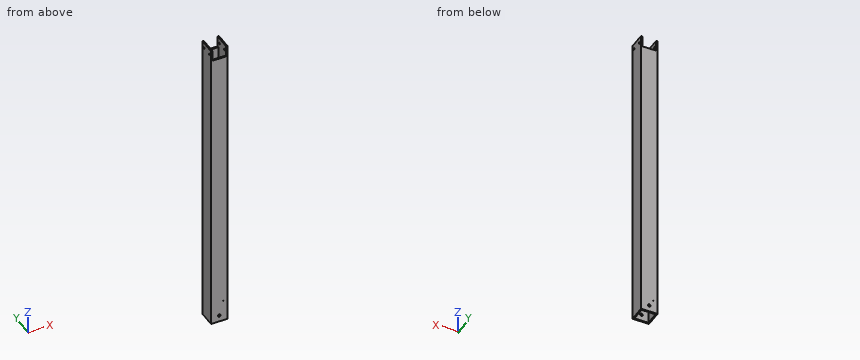
```python
from build123d import *

# Parameters (mm, degrees)
ESQUISSE2_W             = 38.1
ESQUISSE2_H             = 38.1
ESQUISSE2_W_2           = 31.75
ESQUISSE2_H_2           = 31.75
BOSS_EXTRU_1_DEPTH      = 350
ESQUISSE3_R             = 2.159
ENL_V_MAT_EXTRU_1_DEPTH = 353.582632159
ESQUISSE4_W             = 31.75
ESQUISSE4_H             = 25.4
ENL_V_MAT_EXTRU_2_DEPTH = 353.582632159
ESQUISSE6_R             = 3.175
ENL_V_MAT_EXTRU_3_DEPTH = 353.582632159
ESQUISSE8_R             = 0.5
ENL_V_MAT_EXTRU_4_DEPTH = 352.035332979
ESQUISSE8_3_R           = 0.5
ENL_V_MAT_EXTRU_5_DEPTH = 352.035332979


with BuildPart() as part:
    # Esquisse2 → Boss.-Extru.1 (new, symmetric)
    with BuildSketch(Plane.XY):
        Rectangle(ESQUISSE2_W, ESQUISSE2_H)
        Rectangle(ESQUISSE2_W_2, ESQUISSE2_H_2, mode=Mode.SUBTRACT)
    extrude(amount=BOSS_EXTRU_1_DEPTH, both=True)

    # Esquisse3 → Enl_v. mat.-Extru.1 (cut, through all)
    with BuildSketch(Plane.ZY.offset(19.05)):
        with Locations((337.3, -11.43)):
            Circle(ESQUISSE3_R)
    enl_v_mat_extru_1 = extrude(amount=-ENL_V_MAT_EXTRU_1_DEPTH, mode=Mode.SUBTRACT)

    # Sym_trie1: Enl_v. mat.-Extru.1 across plane
    add(enl_v_mat_extru_1.mirror(Plane.ZX), mode=Mode.SUBTRACT)

    # Esquisse4 → Enl_v. mat.-Extru.2 (cut, through all)
    with BuildSketch(Plane.XZ.offset(19.05)):
        with Locations((0, 337.3)):
            Rectangle(ESQUISSE4_W, ESQUISSE4_H)
    extrude(amount=-ENL_V_MAT_EXTRU_2_DEPTH, mode=Mode.SUBTRACT)

    # Esquisse6 → Enl_v. mat.-Extru.3 (cut, through all)
    with BuildSketch(Plane.XZ.offset(19.05)):
        with Locations(Location((0, -335, 0), (0, 0, 270))):
            Circle(ESQUISSE6_R)
    extrude(amount=-ENL_V_MAT_EXTRU_3_DEPTH, mode=Mode.SUBTRACT)

    # Esquisse8 → Enl_v. mat.-Extru.4 (cut, through all)
    with BuildSketch(Plane(origin=(0, 0, 0), x_dir=(1, 0, 0), z_dir=(0, 1, 0))):
        with Locations(Location((9.525, 320, 0), (0, 0, 270))):
            Circle(ESQUISSE8_R)
        with Locations(Location((9.525, 300, 0), (0, 0, 270))):
            Circle(ESQUISSE8_R)
    extrude(amount=-ENL_V_MAT_EXTRU_4_DEPTH, mode=Mode.SUBTRACT)

    # Esquisse8_3 → Enl_v. mat.-Extru.5 (cut, through all)
    with BuildSketch(Plane(origin=(0, 0, 0), x_dir=(1, 0, 0), z_dir=(0, 1, 0))):
        with Locations(Location((-9.525, 300, 0), (0, 0, 90))):
            Circle(ESQUISSE8_3_R)
        with Locations(Location((-9.525, 320, 0), (0, 0, 90))):
            Circle(ESQUISSE8_3_R)
    extrude(amount=ENL_V_MAT_EXTRU_5_DEPTH, mode=Mode.SUBTRACT)


solid = part.part
```
Build history of the part. All positions in model axes, mm. Round coordinates to 2 decimals unless told otherwise and drop trailing zeros. Write each loop counter-clockwise with the first axis right and the second up, starting at its lowest first coordinate (ties: lowest second). Pieces come first, ordered by that corner, then holes. Notation, with made-up numbers: (-9.75, -9) - (44.25, -9) arc R28 cw to (44.25, 15) - close; hole circle Ø6 at (18, -29.5). An arc over 180 degrees is marked (long way). Write each question's results on one line, items separated by ' | '. Start each with the question number.
Item 1: Drop flat-ended pins along their axis: P1, Ø2.5, axis at y = -11.43, z = 337.3, coming from the +X side; P2, Ø2.5, axis at x = -2, y = 17, coming from the +Z side. Give the stop position or say it passes through.
Item 2: Saw through at B-B (z = 182.5). Write the cut outline in (x, y) (3 decimals), and give its area (3 significant figures).
Item 3: Wall check: L1, parallel to Y at x = 17, z = 337.3; L2, parallel to X at y = 3.5, z = 196 (3 decimals); L3, parallel to X at y = -17.65, z = -335 (3 decimals). Give the ranges that are in metal, low to high. Write a range as [from, to].
Item 4: Saw through at A-A (y = 1.5). Write the cut outline in (x, z) (3 decimals).
Results are:
1) P1: passes through | P2: stops at z = 324.6
2) outline: (-19.05, -19.05) - (19.05, -19.05) - (19.05, 19.05) - (-19.05, 19.05) - close; hole (-15.875, -15.875) - (15.875, -15.875) - (15.875, 15.875) - (-15.875, 15.875) - close | area: 444 mm²
3) L1: y = [-19.05, -13.59], [-9.27, 9.27], [13.59, 19.05] | L2: x = [-19.05, -15.875], [15.875, 19.05] | L3: x = [-19.05, -3.175], [3.175, 19.05]
4) outline: (-19.05, -350) - (-15.875, -350) - (-15.875, 350) - (-19.05, 350) - close; (15.875, -350) - (19.05, -350) - (19.05, 350) - (15.875, 350) - close
